Model file for the job. Use its own axes, mm. A direction names the side the tool comes from. Coordinates: 2 decimals unless noted, no trailing zeros. Order: outer loops, then holes, each group sorted by start corner. A loop starts at its lowest first (then second) coordinate and runs counter-clockwise, first axis right, second up. Notation, with made-up numbers: (19, -20.5) -> (51, -20.5) arc R31 ccw to (51, 13.5) -> close; hole circle Ø6 at (-33, 74). An arc over 180 degrees is marked (long way). Write item = value, one per line. Start each with the question number.
Q1. Cut at A-A, the plane z = -47.5. List the corners of the cut face in (x, y).
Q2. Wall check: line 1 (Z direction, x = 54.5, y = 5.25); line 2 (X direction, y = 2.75, z = -55.5); line 3 (Y direction, x = 72, z = -60). Give the ranges that are in metal, low to high. Write a range as from..to.
Q3. Cut at C-C, the plane x = 58. List the corners of the cut face in (y, z), plus the area to 3 significant figures.
Q4. 3-axis set-ups, long thin cutter, end or side, ignore diameter. For faces 1 (the face through (7, 5, -1)), 2 (the face through (0, 5, -32)): which of +Z, -Z, +X, -X, +Y, -Y reach the whole face in a straight line?
Q5. Mould opens along Y. For faces 3 (the face through (1, 5, -57)), 4 (the face through (2.124, 5, -32)), 5 (the face through (140.337, 5, -31)), 6 (the face through (69.8, 10, -57.2)) say: +Y half, -Y half, draft (parallel to the pull), parting line (faces both ways), or undercut.
from build123d import *

# Parameters (mm, degrees)
SKETCH7_W           = 120.227524024
SKETCH7_H           = 41.502027866
BOSS_EXTRUDE4_DEPTH = 10
SKETCH9_W           = 60.894825735
SKETCH9_H           = 8
CUT_EXTRUDE4_DEPTH  = 9
SKETCH12_W          = 60.894825735
SKETCH12_H          = 8
CUT_EXTRUDE6_DEPTH  = 8
SKETCH14_W          = 138.336754021
SKETCH14_H          = 8
CUT_EXTRUDE7_DEPTH  = 9
SKETCH17_W          = 138.336754021
SKETCH17_H          = 8
CUT_EXTRUDE8_DEPTH  = 9
SKETCH20_W          = 128.336754021
SKETCH20_H          = 50.894825735
CUT_EXTRUDE10_DEPTH = 10


with BuildPart() as part:
    # Sketch7 → Boss-Extrude4 (new body)
    with BuildSketch(Plane(origin=(0, 0, 0), x_dir=(1, 0, 0), z_dir=(0, 1, 0))):
        Polygon((0, 0), (11.124254892, 0), (131.351778916, 0), (140.336754021, 0), (140.336754021, 62.894825735), (131.351778916, 62.894825735), (11.124254892, 62.894825735), (0, 62.894825735), align=None)
        with Locations((71.238016904, 32.303124782)):
            Rectangle(SKETCH7_W, SKETCH7_H, mode=Mode.SUBTRACT)
    extrude(amount=BOSS_EXTRUDE4_DEPTH)

    # Sketch9 → Cut-Extrude4 (cut)
    with BuildSketch(Plane(origin=(11.124254892, 0, 0), x_dir=(0, 0, -1), z_dir=(1, 0, 0))):
        with Locations((31.447412868, 5)):
            Rectangle(SKETCH9_W, SKETCH9_H)
    extrude(amount=-CUT_EXTRUDE4_DEPTH, mode=Mode.SUBTRACT)

    # Sketch12 → Cut-Extrude6 (cut)
    with BuildSketch(Plane.ZY.offset(-131.351778916)):
        with Locations((-31.447412868, 5)):
            Rectangle(SKETCH12_W, SKETCH12_H)
    extrude(amount=-CUT_EXTRUDE6_DEPTH, mode=Mode.SUBTRACT)

    # Sketch14 → Cut-Extrude7 (cut)
    with BuildSketch(Plane.XY.offset(-53.054138715)):
        with Locations((70.168377011, 5)):
            Rectangle(SKETCH14_W, SKETCH14_H)
    extrude(amount=-CUT_EXTRUDE7_DEPTH, mode=Mode.SUBTRACT)

    # Sketch17 → Cut-Extrude8 (cut)
    with BuildSketch(Plane(origin=(0, 0, -11.552110849), x_dir=(-1, 0, 0), z_dir=(0, 0, -1))):
        with Locations((-70.168377011, 5)):
            Rectangle(SKETCH17_W, SKETCH17_H)
    extrude(amount=-CUT_EXTRUDE8_DEPTH, mode=Mode.SUBTRACT)

    # Sketch20 → Cut-Extrude10 (cut)
    with BuildSketch(Plane(origin=(0, 10, 0), x_dir=(1, 0, 0), z_dir=(0, 1, 0))):
        with Locations((70.168377011, 31.447412868)):
            Rectangle(SKETCH20_W, SKETCH20_H)
    extrude(amount=-CUT_EXTRUDE10_DEPTH, mode=Mode.SUBTRACT)


solid = part.part
Here are the results:
q1.outline = (0, 0) -> (6, 0) -> (6, 1) -> (2.12, 1) -> (2.12, 9) -> (6, 9) -> (6, 10) -> (0, 10) -> close; (134.34, 0) -> (140.34, 0) -> (140.34, 10) -> (134.34, 10) -> (134.34, 9) -> (139.35, 9) -> (139.35, 1) -> (134.34, 1) -> close
q2.line_1 = -62.89..-62.05, -2.55..0
q2.line_2 = 0..1, 139.35..140.34
q2.line_3 = 0..1, 9..10
q3.outline = (0, -62.89) -> (10, -62.89) -> (10, -56.89) -> (9, -56.89) -> (9, -62.05) -> (1, -62.05) -> (1, -56.89) -> (0, -56.89) -> close; (0, -6) -> (1, -6) -> (1, -2.55) -> (9, -2.55) -> (9, -6) -> (10, -6) -> (10, 0) -> (0, 0) -> close
q3.area = 51.1 mm²
q4.face_1 = none
q4.face_2 = +Z, -Z, -X, +Y, -Y
q5.face_3 = undercut
q5.face_4 = undercut
q5.face_5 = draft
q5.face_6 = +Y half
